Autodesk Inventor part; units mm, degrees
ref_plane "Work Plane1" through (0, -10, 0) normal (0, 0, -1) x (0, 1, 0)
ref_plane "Work Plane3" through (0, 0, 0.45) normal (-1, 0, 0) x (0, 1, 0)
ref_plane "YZ Plane" through (0, 0, 0) normal (1, 0, 0) x (0, 1, 0)
sketch "Skizze1" plane through (0, 0, 0) normal (0, 1, 0) x (-1, 0, 0)
  arc A0 (-1.9024, 0.878) -> (-1.9024, -0.878) centre (-2.1, 0) ccw
  arc A1 (-2.0036, 0.4395) -> (-2.0036, -0.4395) centre (-2.1, 0) ccw
  line L0 (0, 0.45) -> (2, 0.45)
  line L1 (0, -0.45) -> (2, -0.45)
  line L2 (2, 0.45) -> (6, 1.9825)
  line L3 (6, 1.9825) -> (6.1503, 1.5901)
  line L4 (6.1503, 1.5901) -> (2, 0)
  line L5 (2, 0) -> (7.7503, -2.2031)
  line L6 (7.7503, -2.2031) -> (7.6, -2.5955)
  line L7 (7.6, -2.5955) -> (2, -0.45)
  line L8 (0, 0) -> (-2.0036, -0.4395)
  line L9 (0, 0) -> (-2.0036, 0.4395)
  line L10 (0, 0.45) -> (0, -0.45) construction
  line L11 (0, 0.45) -> (-1.9024, 0.878)
  line L12 (0, -0.45) -> (-1.9024, -0.878)
  line L13 (-3, 0) -> (2, 0) construction
  line L14 (2, 0.45) -> (2, -0.45) construction
  dimension "d0" = 2
  dimension "d1" = 6
  dimension "d2" = 159.037
  dimension "d3" = 159.037
  dimension "d4" = 1.6
  dimension "d5" = 0.45
  dimension "d6" = 0.9
  dimension "d7" = 0.45
  dimension "d8" = 0.45
  dimension "d9" = 2.1
extrude "Körper" add sketch "Skizze1" along normal mid plane 0.9
fillet "Rundung" radius 0.315 14 edges at (-4, -0.45, 1.2162) (-4, 0.45, 1.2162) (-1, -0.45, 0.45) (-1, 0.45, 0.45) (3, -0.45, 0) (0.9512, -0.45, -0.664) (0.9512, -0.45, 0.664) (3, 0.45, 0) (0.9512, 0.45, 0.664) (0.9512, 0.45, -0.664) (-1, -0.45, -0.45) (-4.8, -0.45, -1.5227) (-1, 0.45, -0.45) (-4.8, 0.45, -1.5227)
ref_plane "Work Plane1" through (0, -10, 0) normal (0, 0, -1) x (0, 1, 0)
ref_plane "Work Plane3" through (0, 0, 0.45) normal (-1, 0, 0) x (0, 1, 0)
equation "\"d0\" = MSIAB"
equation "\"d1\" = SNLG"
equation "\"d4\" = LGDIF"
equation "\"d5\" = -0.5 * SNND1 + 0.5 * KBR"
equation "\"d6\" = 0.5 * KBR"
equation "\"d7\" = 0.5 * SNND1"
equation "\"d8\" = 0.5 * SNND1"
equation "\"d9\" = KOL - 0.5 * KBR"
equation "\"d10\" = SNND1"
equation "\"d12\" = 0.35 * SNND1"
equation "\"SNND\" = 1"
equation "\"SNLG\" = 6"
equation "\"SNND1\" = 0.9"
equation "\"KBR\" = 1.8"
equation "\"KOL\" = 3"
equation "\"LGDIF\" = 1.6"
equation "\"MSIAB\" = 2"
equation "\"BDMI\" = 3"
equation "\"NNDMIN\" = 3.5"
equation "\"SPBOR\" = SNND"
equation "\"DSH\" = 2.2"
equation "\"NNDMAX\" = 4.5"
equation "\"PNDST\" = 4"
equation "\"BDMA\" = 4"
properties part number "DIN 94 - 1 x 6" material "Stahl, weich"
Part model, mm, in its own coordinate system. A direction names the side the tool comes from. Round coordinates to 2 decimals unless told otherwise and drop trailing zeros. Loops run counter-clockwise (first coordinate to the right, second up) from the corner with the lowest first, then second, coordinate; pieces in that order, holes last. Notation, with made-up numbers: (-37, 53) - (-20, 53) arc R20 cw to (-20, 81) - close; hole circle Ø3 at (-2.75, -16). An arc over 180 degrees is marked (long way). Answer as a JSON object with one key per item and string values.
Item 1: Pull direction X, two halves, no side cores. Call faces 5 (the face through (-4.835, -0.006, -1.086)), 6 (the face through (2.55, -0.01, -0.01)), 7 (the face through (-4.04, -0.36, 1.13)): pulls with the +X half, pulls with the -X half, needs draft (parallel to the pull), parting line crosses it, or undercut.
Output:
{"face 5": "pulls with the -X half", "face 6": "undercut", "face 7": "undercut"}
Item 2: Band-saw the part on A-A on y = 0. List the corners of the cut face in (x, z), plus the area to 3 significant figures.
Output:
{"outline": "(-7.75, -2.2) - (-7.6, -2.6) - (-2, -0.45) - (0, -0.45) - (1.9, -0.88) arc R0.9 ccw (long way) to (1.9, 0.88) - (0, 0.45) - (-2, 0.45) - (-6, 1.98) - (-6.15, 1.59) - (-2, 0) - close; hole (0, 0) - (2, -0.44) arc R0.45 ccw (long way) to (2, 0.44) - close", "area": "9.05 mm2"}
Item 3: Tool access for faces 1 (the face through (-4.033, 0.355, 1.133)), 2 (the face through (-4.104, -0.006, 0.806)), 3 (the face through (0.988, -0.006, 0.217)), 4 (the face through (-4.77, -0.36, -1.41)): list every direction of +Z, -Z, +X, -X, +Y, -Y with a clear straight run to the whole face (end or side of a thin tool).
Output:
{"face 1": "+Z, +Y", "face 2": "-X, +Y, -Y", "face 3": "+Y, -Y", "face 4": "-Z, -Y"}
Item 4: Wall check: L1, parallel to Z at x = 2.1, y = -0.05; L2, parallel to Z at x = -5, y = 0; L3, parallel to Y at x = 0.25, z = 0.25. Give the ranges that are in metal, low to high.
Output:
{"L1": "-0.9 to -0.45, 0.45 to 0.9", "L2": "-1.6 to -1.15, 1.15 to 1.6", "L3": "-0.44 to 0.44"}
Item 5: Band-saw the part on B-B on x = 2.1. List the corners of the cut face in (y, z) (3 decimals).
Output:
{"outline": "(-0.45, -0.585) arc R0.315 ccw to (-0.135, -0.9) - (0.135, -0.9) arc R0.315 ccw to (0.45, -0.585) - (0.45, -0.45) - (-0.45, -0.45) - close; (-0.45, 0.45) - (0.45, 0.45) - (0.45, 0.585) arc R0.315 ccw to (0.135, 0.9) - (-0.135, 0.9) arc R0.315 ccw to (-0.45, 0.585) - close"}
